Geometry: see drawing. Coordinates: mm, zero at the bounding-box minimum. Coordinates: 2 decimals unless noted, no trailing zeros. Write each loop counter-clockwise with the first axis right and the second up, starting at its lowest first coordinate (ties: lowest second). Pieces come first, ordered by that corner, then holes. Notation, with made-up numbers: M 53.5,43.25 L 69.5,43.25 A17 cw 69.5,55.25 Z; hole C 76.25,51.25 d9. An arc over 180 degrees is marked long. One line per item, written item: value. Start each with the question number.
Item 1: Pin query (flat end, axial travel): P1, Ø10, axis at x = 144.5, y = 27.5, coming from the -Z side; P2, Ø0.9, axis at y = 37, z = 2, coming from the -X side; P3, Ø1.5, axis at x = 170.5, z = 1.5, coming from the -Y side; P4, Ø1.5, axis at x = 45, z = 2, coming from the +Y side. Return the tip coordinate at first contact, or that it passes through.
Item 2: Cut plane A-A, the plane x = 134. Output: boundary loops of the cut face in (y, z).
Item 3: Ray query, L1, parallel to X at y = 2, z = 2.25; L2, parallel to X at y = 36, z = 2.55; L3, parallel to Y at x = 60.5, z = 1.6. Return the intervals inside material, ascending. Write a range as from..to.
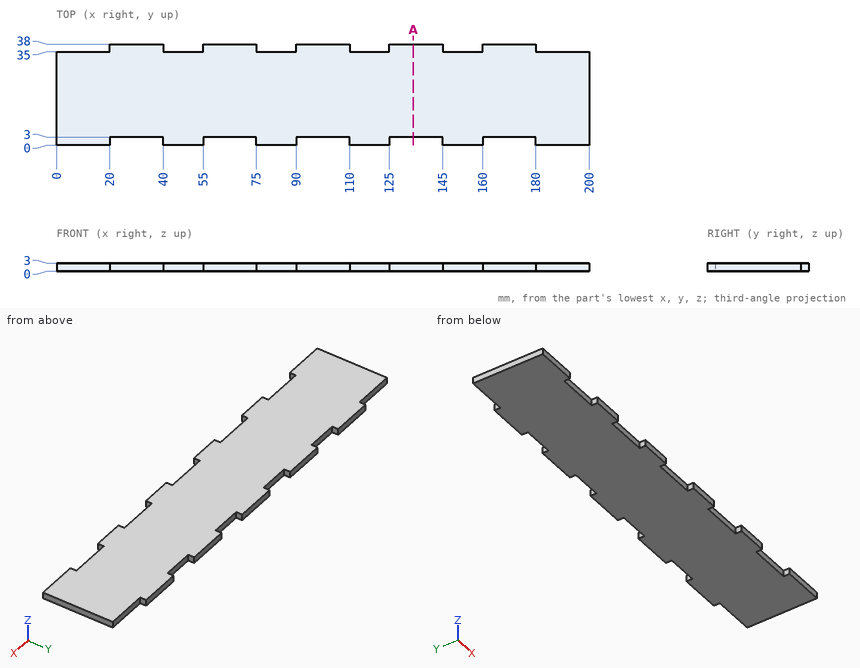
From the geometry:
1. P1: stops at z = 0
1. P2: stops at x = 20
1. P3: stops at y = 3
1. P4: stops at y = 35
2. outline: M 3,0 L 38,0 L 38,3 L 3,3 Z
3. L1: x = 0..20, 40..55, 75..90, 110..125, 145..160, 180..200
3. L2: x = 20..40, 55..75, 90..110, 125..145, 160..180
3. L3: y = 3..38
